Autodesk Inventor part; units mm, degrees
ref_plane "IP_dummy_XY" through (0, 0, 0) normal (1, 0, 0) x (0, 0, -1)
ref_plane "IP_dummy_YZ" through (0, 0, 0) normal (0, 0, -1) x (0, 1, 0)
ref_plane "IP_dummy_ZX" through (0, 0, 0) normal (0, 1, 0) x (1, 0, 0)
sketch "Sketch_1" plane through (0, 0, 0) normal (0, 0, 1) x (1, 0, 0)
  line L0 (36, 0) -> (0, 0)
  line L1 (0, 0) -> (0, 9.92)
  line L2 (0, 9.92) -> (0.48, 10.4)
  line L3 (0.48, 10.4) -> (1.6, 10.4)
  line L4 (1.6, 10.4) -> (1.6, 10.8333)
  line L5 (1.6, 10.8333) -> (0.4, 10.8333)
  line L6 (0.4, 10.8333) -> (0.4, 12.7)
  arc A0 (0.7, 13) -> (0.4, 12.7) centre (0.7, 12.7) ccw
  line L7 (0.7, 13) -> (12.1, 13)
  arc A1 (12.4, 12.7) -> (12.1, 13) centre (12.1, 12.7) ccw
  line L8 (12.4, 12.7) -> (12.4, 10.8333)
  line L9 (12.4, 10.8333) -> (11.2, 10.8333)
  line L10 (11.2, 10.8333) -> (11.2, 10.4)
  line L11 (11.2, 10.4) -> (12.52, 10.4)
  line L12 (12.52, 10.4) -> (13, 9.92)
  line L13 (13, 9.92) -> (13, 5)
  line L14 (13, 5) -> (35.08, 5)
  line L15 (35.08, 5) -> (36, 4.08)
  line L16 (36, 4.08) -> (36, 0)
  line L17 (36, 0) -> (0, 0)
revolve "Revolution1" add sketch "Sketch_1" angle 360 about axis through (36, 0, 0) along (1, 0, 0)
thread "Thread1"
sketch "Sketch2" plane through (0, 0, 0) normal (-1, 0, 0) x (0, 0, 1)
  point P0 (0, 0)
hole "Hole1" at (0, 0, 0) direction (1, 0, 0) diameter 4 depth 5.2 tip angle 113.952
sketch "Sketch_5" plane through (0, 0, 0) normal (0, 1, 0) x (-1, 0, 0)
  arc A0 (0, 5.5) -> (-1.375, 2.5) centre (6.4286, 0.7384) ccw
  line L0 (-1.375, 2.5) -> (-1.375, -2.5)
  arc A1 (-1.375, -2.5) -> (0, -5.5) centre (6.4286, -0.7384) ccw
  line L1 (0, -5.5) -> (0, 5.5)
extrude "Extrusion1" cut sketch "Sketch_5" along normal mid plane 1.5
ref_plane "IP_dummy_XY" through (0, 0, 0) normal (1, 0, 0) x (0, 0, -1)
ref_plane "IP_dummy_YZ" through (0, 0, 0) normal (0, 0, -1) x (0, 1, 0)
ref_plane "IP_dummy_ZX" through (0, 0, 0) normal (0, 1, 0) x (1, 0, 0)
ref_plane "IP_grease_nipple_XY" through (0, 0, 0) normal (1, 0, 0) x (0, 0, -1)
ref_plane "IP_grease_nipple_YZ" through (0, 0, 0) normal (0, 0, -1) x (0, 1, 0)
ref_plane "IP_grease_nipple_ZX" through (0, 0, 0) normal (0, 1, 0) x (1, 0, 0)
properties part number "CAM FOLLOWER"
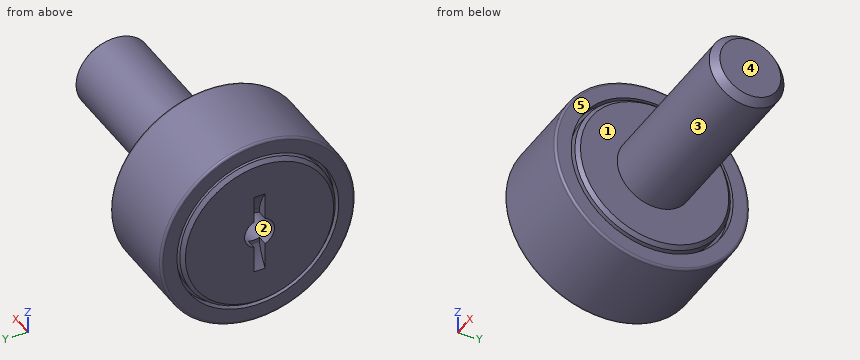
Verification items for the finished model (mm, model axes). Face numbers are marked on the shaded views. A direction names the side the tool comes from. Give positions to 0.01 mm unless a question says otherwise; leave off trailing zeros. Order: outer loops, then holes, each group sorted by start corner. A loop starts at its lowest first (then second) coordinate and runs counter-clockwise, first axis right, second up. Notation, with made-up numbers: (65, 11) -> (87, 11) arc R18 cw to (87, 44) -> close; hole circle Ø9 at (2, 9.25). An arc over 180 degrees is marked (long way). Answer as CSV lines item,"result".
Q1. Sectioned sample at A-A on x = 7.5. Record the cut outline in (y, z), plus the area to 3 significant figures.
Solutions:
outline,"circle Ø26 at (0, 0)"
area,"531 mm²"
Q2. Depth check by flat-ended pin: pin 1 (12 mm diameter, centred on x = 30, y = 8, fed in from -Z); pin 2 (1.1 mm diameter, centred on x = 1, z = 3.5, fed in from +Y); pin 3 (12 mm diameter, centred on x = 32, z = 5, fed in from -Y). Enter the tip coordinate at first touch or a pass-through.
Solutions:
pin 1,"stops at z = -4.58"
pin 2,"stops at y = 12.66"
pin 3,"stops at y = -5"
Q3. Scan lines: probe 1 along X at (y, z) = (-6.5, -7.5); probe 2 along X at (y, z) = (-2.5, 11.75); probe 3 along Y at (x, z) = (10, -8.25). Record each from-to range of solid material in increasing order.
Solutions:
probe 1,"x = 0 to 13"
probe 2,"x = 0.4 to 12.4"
probe 3,"y = -10.05 to 10.05"
Q4. Access from +Z, -Z, +X, -X, +Y, -Y to the whole of each face (thin tool, end or side, straight path). Record for the marked faces 4 and 5.
Solutions:
face 4,"+Z, -Z, +X, +Y, -Y"
face 5,"+X"
Q5. Release check for a two-part mould opening along Z. For the marked faces 1, 2 and 3 record: +Z half, -Z half, draft (parallel to the pull), parting line (faces both ways), or undercut.
Solutions:
face 1,"draft"
face 2,"undercut"
face 3,"parting line"
Q6. Sectioned sample at B-B on x = 27. Record the cut outline in (y, z), plus the area to 3 significant figures.
Solutions:
outline,"circle Ø10 at (0, 0)"
area,"78.5 mm²"
